Can you work these out from the model? Positions are in its coordinate system, mm. Face numbers are marked on the shaded views. A direction names the side the tool comes from. Give positions to 0.01 mm unless a question says otherwise; leave off trailing zeros. Order: outer loops, then holes, each group sorted by start corner. A loop starts at its lowest first (then second) coordinate and runs counter-clockwise, first axis right, second up. Notation, with made-up numbers: (86, 8.25) -> (91, 8.25) arc R31 cw to (91, 39.25) -> close; hole circle Ø10 at (1.25, 50). An arc over 180 degrees is marked (long way). Answer as a JSON object with one key per item and string values.
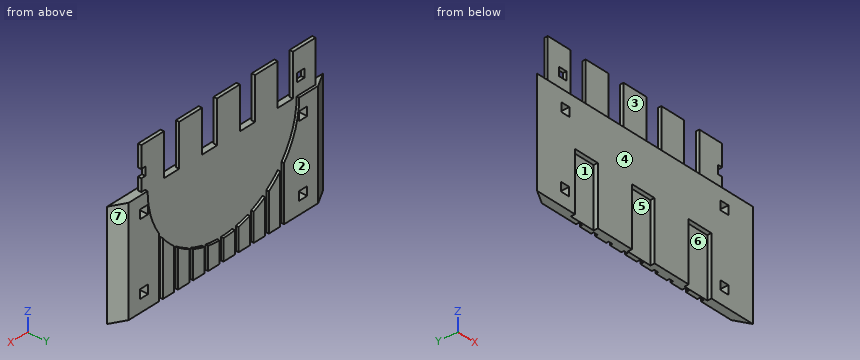
```python
from build123d import *

# Parameters (mm, degrees)
SKETCH_1_W          = 250
SKETCH_1_H          = 125
EXTRUDE_1_DEPTH     = 10
SKETCH_5_W          = 10
SKETCH_5_H          = 10
CUT_EXTRUDE_1_DEPTH = 10
CUT_EXTRUDE_2_DEPTH = 3
SKETCH_8_W          = 30
SKETCH_8_H          = 4
EXTRUDE_2_DEPTH     = 50
SKETCH_11_W         = 10
SKETCH_11_H         = 10
CUT_EXTRUDE_4_DEPTH = 10
CUT_EXTRUDE_5_DEPTH = 3
EXTRUDE_3_DEPTH     = 125
SKETCH_14_W         = 30
SKETCH_14_H         = 69.595930906
CUT_EXTRUDE_6_DEPTH = 5
SKETCH_16_W         = 10.517397933
SKETCH_16_H         = 10.423374962
SKETCH_16_H_2       = 10.423374961
SKETCH_16_W_2       = 10.517397932
CUT_EXTRUDE_7_DEPTH = 190.684282477


with BuildPart() as part:
    # 草图1 → 凸台-拉伸1 (new body)
    with BuildSketch(Plane(origin=(0, 0, 0), x_dir=(1, 0, 0), z_dir=(0, 1, 0))):
        with Locations((0, 62.5)):
            Rectangle(SKETCH_1_W, SKETCH_1_H)
    extrude(amount=EXTRUDE_1_DEPTH)

    # 草图5 → 切除-拉伸1 (cut)
    with BuildSketch(Plane(origin=(0, 10, 0), x_dir=(1, 0, 0), z_dir=(0, 1, 0))):
        with Locations((-105, 105)):
            Rectangle(SKETCH_5_W, SKETCH_5_H)
        with Locations((-105, 20)):
            Rectangle(SKETCH_5_W, SKETCH_5_H)
        with Locations((105, 105)):
            Rectangle(SKETCH_5_W, SKETCH_5_H)
        with Locations((105, 20)):
            Rectangle(SKETCH_5_W, SKETCH_5_H)
    extrude(amount=-CUT_EXTRUDE_1_DEPTH, mode=Mode.SUBTRACT)

    # 草图6 → 切除-拉伸2 (cut)
    with BuildSketch(Plane(origin=(0, 10, 0), x_dir=(1, 0, 0), z_dir=(0, 1, 0))):
        with BuildLine():
            Line((-100, 0), (100, 0))
            ThreePointArc((100, 0), (0, 100), (-100, 0))
        make_face()
    extrude(amount=-CUT_EXTRUDE_2_DEPTH, mode=Mode.SUBTRACT)

    # 草图8 → 凸台-拉伸2 (add)
    with BuildSketch(Plane.XY):
        with Locations((-110, 5)):
            Rectangle(SKETCH_8_W, SKETCH_8_H)
        with Locations((-60, 5)):
            Rectangle(SKETCH_8_W, SKETCH_8_H)
        with Locations((-10, 5)):
            Rectangle(SKETCH_8_W, SKETCH_8_H)
        with Locations((40, 5)):
            Rectangle(SKETCH_8_W, SKETCH_8_H)
        with Locations((90, 5)):
            Rectangle(SKETCH_8_W, SKETCH_8_H)
    extrude(amount=EXTRUDE_2_DEPTH)

    # 草图11 → 切除-拉伸4 (cut)
    with BuildSketch(Plane(origin=(0, 10, 0), x_dir=(1, 0, 0), z_dir=(0, 1, 0))):
        Polygon((104.677013389, -14.646181821), (112.233893295, -14.646181821), (112.233893295, -24.646181821), (104.677013389, -24.646181821), (99.677013389, -24.646181821), (99.677013389, -14.646181821), align=None)
        with Locations((-105.322986611, -19.646181821)):
            Rectangle(SKETCH_11_W, SKETCH_11_H)
    extrude(amount=-CUT_EXTRUDE_4_DEPTH, mode=Mode.SUBTRACT)

    # 草图12 → 切除-拉伸5 (cut)
    with BuildSketch(Plane(origin=(0, 10, 0), x_dir=(1, 0, 0), z_dir=(0, 1, 0))):
        with BuildLine():
            Line((-80, 131.028694586), (-75, 131.028694586))
            Line((-75, 131.028694586), (-75, 66.143782777))
            ThreePointArc((-75, 66.143782777), (-77.560856859, 63.121418578), (-80, 60))
            Line((-80, 60), (-80, 131.028694586))
        make_face()
        with BuildLine():
            Line((85, 131.028694586), (85, 52.678268764))
            ThreePointArc((85, 52.678268764), (82.581183917, 56.394574765), (80, 60))
            Line((80, 60), (80, 131.028694586))
            Line((80, 131.028694586), (85, 131.028694586))
        make_face()
        with BuildLine():
            Line((65, 131.028694586), (65, 75.993420768))
            ThreePointArc((65, 75.993420768), (62.532097112, 78.036765891), (60, 80))
            Line((60, 80), (60, 131.028694586))
            Line((60, 131.028694586), (65, 131.028694586))
        make_face()
        with BuildLine():
            Line((45, 131.028694586), (45, 89.302855497))
            ThreePointArc((45, 89.302855497), (42.516221011, 90.511717202), (40, 91.651513899))
            Line((40, 91.651513899), (40, 131.028694586))
            Line((40, 131.028694586), (45, 131.028694586))
        make_face()
        with BuildLine():
            Line((25, 131.028694586), (25, 96.824583655))
            ThreePointArc((25, 96.824583655), (22.507410108, 97.434164903), (20, 97.979589711))
            Line((20, 97.979589711), (20, 131.028694586))
            Line((20, 131.028694586), (25, 131.028694586))
        make_face()
        with BuildLine():
            Line((5, 131.028694586), (5, 99.874921777))
            ThreePointArc((5, 99.874921777), (2.500782106, 99.968725554), (0, 100))
            Line((0, 100), (0, 131.028694586))
            Line((0, 131.028694586), (5, 131.028694586))
        make_face()
        with BuildLine():
            Line((-15, 131.028694586), (-15, 98.868599666))
            ThreePointArc((-15, 98.868599666), (-17.505644366, 98.455839925), (-20, 97.979589711))
            Line((-20, 97.979589711), (-20, 131.028694586))
            Line((-20, 131.028694586), (-15, 131.028694586))
        make_face()
        with BuildLine():
            Line((-35, 131.028694586), (-35, 93.674969976))
            ThreePointArc((-35, 93.674969976), (-37.513645432, 92.696960071), (-40, 91.651513899))
            Line((-40, 91.651513899), (-40, 131.028694586))
            Line((-40, 131.028694586), (-35, 131.028694586))
        make_face()
        with BuildLine():
            Line((-55, 131.028694586), (-55, 83.516465442))
            ThreePointArc((-55, 83.516465442), (-57.526875305, 81.796446241), (-60, 80))
            Line((-60, 80), (-60, 131.028694586))
            Line((-60, 131.028694586), (-55, 131.028694586))
        make_face()
    extrude(amount=-CUT_EXTRUDE_5_DEPTH, mode=Mode.SUBTRACT)

    # 草图13 → 凸台-拉伸3 (add)
    with BuildSketch(Plane(origin=(0, 0, -125), x_dir=(-1, 0, 0), z_dir=(0, 0, -1))):
        Polygon((125, 10), (125, 0), (142.320508076, 0), align=None)
        Polygon((-125, 10), (-125, 0), (-142.320508076, 0), align=None)
    extrude(amount=-EXTRUDE_3_DEPTH)

    # 草图14 → 切除-拉伸6 (cut)
    with BuildSketch(Plane.XZ):
        with Locations((-77.320508076, -90.202034547)):
            Rectangle(SKETCH_14_W, SKETCH_14_H)
        with Locations((-2.320508076, -90.202034547)):
            Rectangle(SKETCH_14_W, SKETCH_14_H)
        with Locations((72.679491924, -90.202034547)):
            Rectangle(SKETCH_14_W, SKETCH_14_H)
    extrude(amount=-CUT_EXTRUDE_6_DEPTH, mode=Mode.SUBTRACT)

    # 草图16 → 切除-拉伸7 (cut, through all)
    with BuildSketch(Plane(origin=(0, 10, 0), x_dir=(1, 0, 0), z_dir=(0, 1, 0))):
        with Locations((-105.258698967, 104.788312519)):
            Rectangle(SKETCH_16_W, SKETCH_16_H)
        with Locations((104.720979462, 19.822994084)):
            Rectangle(SKETCH_16_W, SKETCH_16_H_2)
        with Locations((-105.154924979, 19.775983857)):
            Rectangle(SKETCH_16_W_2, SKETCH_16_H)
        with Locations((104.744997222, 104.787129461)):
            Rectangle(SKETCH_16_W, SKETCH_16_H)
    extrude(amount=-CUT_EXTRUDE_7_DEPTH, mode=Mode.SUBTRACT)


solid = part.part
```
1. Will these pins go through, and if not, where does the flat tip stop? pin 1 Ø1 at (x, z) = (-15.5, -90.5) entering from -Y; pin 2 Ø2 at (y, z) = (5.5, 33.5) entering from +X; pin 3 Ø0.9 at (y, z) = (9, -106.5) entering from +X.
Worked answers:
{"pin 1": "y = 5", "pin 2": "x = 105", "pin 3": "x = 127.51"}
2. If we section it at C-C on z = -7: Please give me the cut outline in (x, y), then the cut area to 3 significant figures.
Worked answers:
{"outline": "(-142.32, 0) -> (142.32, 0) -> (125, 10) -> (99.75, 10) -> (99.75, 7) -> (-99.75, 7) -> (-99.75, 10) -> (-125, 10) -> close", "area": "2,070 mm²"}
3. If we mould it in two halves opening along X, with no side actions, what happens to the marked faces 4, 5, 6 and 7? For each: +X half, -X half, draft (parallel to the pull), parting line (faces both ways), or undercut.
Worked answers:
{"face 4": "draft", "face 5": "undercut", "face 6": "undercut", "face 7": "+X half"}
4. If we section it at D-D on z = -32: Please give me the cut outline in (x, y).
Worked answers:
{"outline": "(-142.32, 0) -> (142.32, 0) -> (125, 10) -> (94.74, 10) -> (94.74, 7) -> (-94.74, 7) -> (-94.74, 10) -> (-125, 10) -> close"}
5. If we section it at A-A on z = 39: Please give me the cut outline in (x, y), then the cut area to 3 significant figures.
Worked answers:
{"outline": "(-125, 3) -> (-95, 3) -> (-95, 7) -> (-125, 7) -> close; (-75, 3) -> (-45, 3) -> (-45, 7) -> (-75, 7) -> close; (-25, 3) -> (5, 3) -> (5, 7) -> (-25, 7) -> close; (25, 3) -> (55, 3) -> (55, 7) -> (25, 7) -> close; (75, 3) -> (105, 3) -> (105, 7) -> (75, 7) -> close", "area": "600 mm²"}
6. For the marked faces 1, 2 and 3, which set-ups out of +Z, -Z, +X, -X, +Y, -Y let a thin tool reach every point of the face, with its end or its side?
Worked answers:
{"face 1": "-Z, -Y", "face 2": "+Z, -Z, +X, -X, +Y", "face 3": "+Z, +X, -X, -Y"}
7. If we section it at B-B on y = 8.5: Count the separate pieces of the cut face and the enclosed holes in it, then the cut area to 3 significant figures.
Worked answers:
{"separate pieces": "10", "enclosed holes": "4", "area": "13,900 mm²"}
8. Please list where these lines run through material, in increasing order: L1, parallel to X at y = 7.5, z = -86; L2, parallel to X at y = 1, z = -68; L3, parallel to X at y = 5.5, z = 1.
Worked answers:
{"L1": "-129.33 to -80, -75 to -60, -55 to -51.03, 51.03 to 60, 65 to 80, 85 to 129.33", "L2": "-140.59 to -92.32, -62.32 to -17.32, 12.68 to 57.68, 87.68 to 140.59", "L3": "-125 to -95, -75 to -45, -25 to 5, 25 to 55, 75 to 105"}
